Here's how the part is built. I have some questions about the finished solid (model axes, mm). A direction names the side the tool comes from. Coordinates: 2 decimals unless noted, no trailing zeros. Write each loop counter-clockwise with the first axis right and the second up, starting at its lowest first coordinate (ties: lowest second). Pieces come first, ordered by that corner, then holes.
(1) Imagine slicing it at C-C, the plane y = 0. State how many separate pieces and enclosed holes the cut face has, plus the area to 3 significant figures.
(2) Imagine slicing it at B-B, the plane x = 4. List the corners of the cut face in (y, z) for me.
(3) For pin 1 Ø1 at (x, z) = (18, 4) entering from -Y; pin 2 Ø4 at (x, y) = (26, -2.5) entering from +Z; pin 3 Ø6.5 at (y, z) = (4.5, 0.5) entering from -X, each with a flat end and sliding along its axis, tell me the tip position at first contact or that it passes through.
(4) Imagine slicing it at D-D, the plane x = 10. List the corners of the cut face in (y, z) for me.
(5) Thinking about a two-plate mould opening in X: for faces 5 (the conical face through (2.4, -7.2, 5.5)), 6 (the flat face through (18.827, 0, 6)), 7 (the cylindrical face through (-0.34, -1.72, 7.75)), 8 (the flat face through (2.571, 0, -5)), which applies, released by +X, released by -X, zero draft, split by the parting line, or undercut?
(6) Which directions (+Z, -Z, +X, -X, +Y, -Y) give clear straight access to the entire face, cutting with the end or side of a thin tool? Please do faces 1 (the cylindrical face through (28.137, 7.937, -0.073)), 2 (the cylindrical face through (6.65, 4.29, 9.39)), 3 (the cylindrical face through (28.137, -7.937, 0.073)), 4 (the flat face through (18.446, 0, 0)).
(7) Please list where these lines run through material, in increasing order: probe 1 along Z at (x, y) = (17.5, 0); probe 2 along X at (y, z) = (0, 6); probe 3 along Y at (x, z) = (0.5, -2).
Autodesk Inventor part; units mm, degrees
ref_plane "Work Plane1" through (10.5083, 0, 10.922) normal (0, 0, 1) x (1, 0, 0)
ref_plane "YZ Plane" through (0, 0, 0) normal (1, 0, 0) x (0, 1, 0)
ref_plane "XZ Plane" through (0, 0, 0) normal (0, 1, 0) x (-1, 0, 0)
sketch "Sketch1" plane through (0, 0, 0) normal (0, 0, 1) x (1, 0, 0)
  line L0 (0, 0) -> (35.3368, 0)
  line L1 (0, 10.922) -> (1.397, 9.525)
  line L2 (0, 10.922) -> (0.5388, 10.922)
  line L3 (0.5388, 10.922) -> (2.5708, 8.89)
  line L4 (2.5708, 8.89) -> (2.5708, 10.922)
  line L5 (2.5708, 10.922) -> (18.4458, 10.922)
  line L6 (18.4458, 10.922) -> (18.4458, 7.9248)
  line L7 (18.4458, 7.9248) -> (20.7318, 7.9248)
  line L8 (20.7318, 7.9248) -> (20.7318, 7.9375)
  line L9 (20.7318, 7.9375) -> (35.3368, 7.9375)
  line L10 (35.3368, 7.9375) -> (35.3368, 0)
  circle A0 centre (11.3338, 0) radius 4.7625
  circle A1 centre (27.0818, 0) radius 3.175
  line L11 (0, 10.922) -> (0, 0) construction
  line L12 (0.5388, 10.922) -> (2.5708, 10.922) construction
  line L13 (2.5708, 8.89) -> (2.5708, 7.9375) construction
  line L14 (1.397, 9.525) -> (0, 9.525)
  line L15 (0, 9.525) -> (0, 7.9375) construction
  line L16 (2.5708, 7.9375) -> (0, 7.9375)
  line L17 (0, 9.525) -> (0, 7.9375)
  line L18 (2.5708, 7.9375) -> (2.5708, 4.826)
  line L19 (2.5708, 4.826) -> (18.4458, 4.826)
  line L20 (18.4458, 4.826) -> (18.4458, 0)
  line L21 (18.4458, 7.9248) -> (18.4458, 4.826)
  line L22 (35.3368, 4.826) -> (18.4458, 4.826)
  line L23 (0, 9.525) -> (-3.175, 9.525)
  line L24 (-3.175, 9.525) -> (-3.175, 7.9375)
  line L25 (-3.175, 7.9375) -> (0, 7.9375)
  dimension "d1" = 21.844
  dimension "d2" = 9.525
  dimension "d4" = 2.286
  dimension "d5" = 6.35
  dimension "d6" = 8.636
  dimension "d8" = 15.8496
  dimension "d9" = 15.875
  dimension "d10" = 0.381
  dimension "d11" = 45
  dimension "d12" = 15.748
  dimension "d13" = 17.78
  dimension "d14" = 19.05
  dimension "d15" = 15.875
  dimension "d17" = 9.652
  dimension "d18" = 15.875
  dimension "d19" = 9.652
  dimension "d37" = 3.175
  dimension "d38" = 8.255
revolve "Revolution1" add sketch "Sketch1" angle 360 about axis through (0, 0, 0) along (1, 0, 0) picked at (27.874, 1.2084) contours L20 L22 L10 L0 A1 | A1 L0 | L19 L18 L16 L17 L14 L1 L2 L3 L4 L5 L6 L21 | L21 L7 L8 L9 L10 L22 | L25 L24 L23 L17
extrude "Extrusion2" cut sketch "Sketch1" along normal blind 25.4 contours A0 L0 | L0 A0
ref_plane "Work Plane1" through (10.5083, 0, 10.922) normal (0, 0, 1) x (1, 0, 0)
sketch "Sketch2" plane through (10.5083, 0, 10.922) normal (0, 0, 1) x (1, 0, 0)
  line L0 (0.8255, -4.7625) -> (0.8255, 0) construction
  circle A0 centre (0.8255, 0) radius 6.35
  point P0 (-10.5083, 0)
  dimension "d28" = 12.7
  dimension "d29" = 4.7625
extrude "Extrusion3" cut sketch "Sketch2" against normal blind 2.54
sketch "Sketch3" plane through (35.3368, 0, 0) normal (1, 0, 0) x (0, 0, -1)
  circle A0 centre (0, 0) radius 7.9375
  line L0 (-4.826, 6.3019) -> (-4.826, -6.3019)
  line L1 (4.826, 6.3019) -> (4.826, -6.3019)
  dimension "d32" = 9.652
extrude "Extrusion4" cut sketch "Sketch3" against normal blind 16.51 contours A0 L1 | L0 A0
extrude "Extrusion5" cut sketch "Sketch1" along normal through all both and the other way through all contours A1 L0 | L0 A1
thread "Thread1"
thread "Thread2"
equation "\"d17\" = d19"
properties part number "Rebuild Shooter NCDME075-0600 Cylinder Back Section" material "Aluminum 6061"
Recorded:
1. separate pieces: 3
1. enclosed holes: 0
1. area: 251 mm2
2. outline: circle Ø21.84 at (0, 0); hole circle Ø9.65 at (0, 0)
3. pin 1: stops at y = -10.35
3. pin 2: stops at z = 4.83
3. pin 3: stops at x = 2.57
4. outline: (-6.21, 8.38) - (-6.21, 8.99) arc R10.92 ccw (long way) to (6.21, 8.99) - (6.21, 8.38) - (4.57, 8.38) - (4.57, 1.55) arc R4.83 cw (long way) to (-4.57, 1.55) - (-4.57, 8.38) - close
5. face 5: undercut
5. face 6: released by +X
5. face 7: zero draft
5. face 8: released by -X
6. face 1: +X, +Y
6. face 2: +Z
6. face 3: +X, -Y
6. face 4: -X
7. probe 1: z = -10.92 to -4.83, 4.83 to 8.38
7. probe 2: x = 2.57 to 6.57, 16.1 to 18.83
7. probe 3: y = -10.74 to -10.23, -9.31 to -7.68, 7.68 to 9.31, 10.23 to 10.74
